Geometry: final body of the model. Coordinates: model frame, mm. Face numbers are marked on the shaded views. A direction names the side the tool comes from. Give positions to 0.01 mm unless a question says otherwise; leave off trailing zeros. Order: outer loops, then holes, each group sorted by start corner. A loop starts at its lowest first (then second) coordinate and runs counter-clockwise, first axis right, second up. Notation, with made-up numbers: (-9.75, -8) - (24.25, -8) arc R12 cw to (24.25, 0) - close; hole circle Ø9 at (13.25, 55.5). An arc over 180 degrees is marked (long way). Put each result on its own line as item: value. Start each with the question number.
1. Ray query, line 1 along Z through (x, y) = (-4, 16.5); line 2 along X through (y, z) = (12, -33); line 3 along X through (y, z) = (17, -17.5). Return the intervals inside material, ascending. Write a range as from..to.
2. Section A-A on x = 0. Return the cut outline in (y, z), plus the area to 3 significant figures.
3. Mould query, pull axis Z, two halves, no side actions, for the marked faces 5, 6 and 7. Classes: pulls with the +Z half, pulls with the -Z half, needs draft (parallel to the pull), parting line crosses it, or undercut.
4. First-contact query: P1, Ø3, axis at y = 14.5, z = -39, coming from the +X side; P2, Ø3.5, axis at y = 11, z = 25.59, coming from the -X side; P3, Ø6.5, axis at y = 8.5, z = 25, coming from the +X side. Flat tips, straight axial feed; report the tip coordinate or a pass-through.
5. Section B-B on z = 0. Return the cut outline in (x, y).
6. Set-up query: the marked faces 1, 2, 3 and 4. Return all of +Z, -Z, +X, -X, +Y, -Y with unobstructed straight access to the full face (end or side cutting, diameter ignored); none if empty.
7. Section C-C on y = 17.5. Return the cut outline in (x, z), plus the area to 3 significant figures.
8. Section D-D on y = 11. Count the separate pieces of the cut face and the enclosed holes in it, plus the area to 3 significant figures.
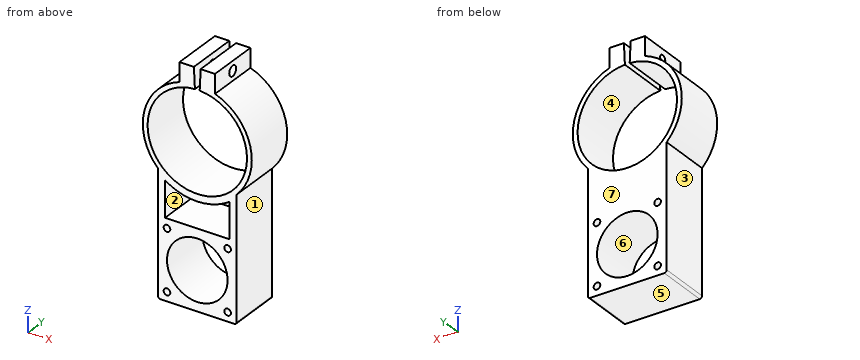
from build123d import *

# Parameters (mm, degrees)
BOSS_EXTRUDE1_DEPTH = 22
CUT_EXTRUDE1_REACH  = 79.458
SKETCH4_R           = 1.5875
CUT_EXTRUDE2_REACH  = 79.458
SKETCH5_R           = 2.159
SKETCH7_R           = 12.7
CUT_EXTRUDE3_DEPTH  = 75.871591195
SKETCH8_R           = 1.397
CUT_EXTRUDE4_DEPTH  = 75.871591195
CUT_EXTRUDE5_DEPTH  = 19
FILLET1_R           = 1


with BuildPart() as part:
    # Sketch1 → Boss-Extrude1 (new body)
    with BuildSketch(Plane(origin=(0, 0, 0), x_dir=(1, 0, 0), z_dir=(0, 1, 0))):
        with BuildLine():
            Line((1, -20.803980004), (1.422212938, -29.587689527))
            Line((1.422212938, -29.587689527), (7.422212938, -29.587689527))
            Line((7.422212938, -29.587689527), (7.422212938, -21.587689527))
            ThreePointArc((7.422212938, -21.587689527), (22.182667824, -5.389511316), (16.5, 15.775537519))
            Line((16.5, 15.775537519), (16.5, 67.828))
            Line((16.5, 67.828), (-16.5, 67.828))
            Line((-16.5, 67.828), (-16.5, 15.775537519))
            ThreePointArc((-16.5, 15.775537519), (-22.182667824, -5.389511316), (-7.422212938, -21.587689527))
            Line((-7.422212938, -21.587689527), (-7.422212938, -29.587689527))
            Line((-7.422212938, -29.587689527), (-1.422212938, -29.587689527))
            Line((-1.422212938, -29.587689527), (-1, -20.803980004))
            ThreePointArc((-1, -20.803980004), (0, 20.828), (1, -20.803980004))
        make_face()
    extrude(amount=BOSS_EXTRUDE1_DEPTH)

    # Cut-Extrude1: up to this plane
    cut_extrude1_end = Plane(origin=(-1, 22, 20.803980004), z_dir=(-0.9988467449508261, 0, -0.04801229114653368))
    # Sketch4 → Cut-Extrude1 (cut, up to the surface)
    with BuildSketch(Plane.ZY.offset(7.422212938), mode=Mode.PRIVATE) as cut_extrude1_sk1:
        with Locations((25.587689527, 11)):
            Circle(SKETCH4_R)
    cut_extrude1_tool1 = split(extrude(cut_extrude1_sk1.sketch, amount=-CUT_EXTRUDE1_REACH, mode=Mode.PRIVATE), bisect_by=cut_extrude1_end, keep=Keep.BOTH, mode=Mode.PRIVATE)
    add(cut_extrude1_tool1.solids().sort_by_distance((-7.422213, 11, 25.58769))[0], mode=Mode.SUBTRACT)

    # Cut-Extrude2: up to this plane
    cut_extrude2_end = Plane(origin=(1, 22, 20.803980004), z_dir=(0.9988467449508261, 0, -0.04801229114653392))
    # Sketch5 → Cut-Extrude2 (cut, up to the surface)
    with BuildSketch(Plane(origin=(7.422212938, 0, 0), x_dir=(0, 0, -1), z_dir=(1, 0, 0)), mode=Mode.PRIVATE) as cut_extrude2_sk1:
        with Locations((-25.587689527, 11)):
            Circle(SKETCH5_R)
    cut_extrude2_tool1 = split(extrude(cut_extrude2_sk1.sketch, amount=-CUT_EXTRUDE2_REACH, mode=Mode.PRIVATE), bisect_by=cut_extrude2_end, keep=Keep.BOTH, mode=Mode.PRIVATE)
    add(cut_extrude2_tool1.solids().sort_by_distance((7.422213, 11, 25.58769))[0], mode=Mode.SUBTRACT)

    # Sketch7 → Cut-Extrude3 (cut, through all)
    with BuildSketch(Plane.XZ):
        with Locations(Location((0, -51.328, 0), (0, 0, 270))):
            Circle(SKETCH7_R)
    extrude(amount=-CUT_EXTRUDE3_DEPTH, mode=Mode.SUBTRACT)

    # Sketch8 → Cut-Extrude4 (cut, through all)
    with BuildSketch(Plane(origin=(0, 22, 0), x_dir=(1, 0, 0), z_dir=(0, 1, 0))):
        with Locations(Location((12.7, 64.028, 0), (0, 0, 270))):
            Circle(SKETCH8_R)
        with Locations(Location((12.7, 38.628, 0), (0, 0, 270))):
            Circle(SKETCH8_R)
        with Locations(Location((-12.7, 38.628, 0), (0, 0, 270))):
            Circle(SKETCH8_R)
        with Locations(Location((-12.7, 64.028, 0), (0, 0, 270))):
            Circle(SKETCH8_R)
    extrude(amount=-CUT_EXTRUDE4_DEPTH, mode=Mode.SUBTRACT)

    # Sketch9 → Cut-Extrude5 (cut)
    with BuildSketch(Plane.XZ):
        with BuildLine():
            Line((-13.5, -34.628), (13.5, -34.628))
            Line((13.5, -34.628), (13.5, -19.634754493))
            ThreePointArc((13.5, -19.634754493), (0, -23.828), (-13.5, -19.634754493))
            Line((-13.5, -19.634754493), (-13.5, -34.628))
        make_face()
    extrude(amount=-CUT_EXTRUDE5_DEPTH, mode=Mode.SUBTRACT)

    # Fillet1
    fillet1_edges = [part.edges().sort_by_distance(p)[0] for p in [
        (-16.5, 11, -67.828),
        (16.5, 11, -67.828),
    ]]
    fillet(fillet1_edges, radius=FILLET1_R)


solid = part.part
Resolved:
1. line 1: -67.83..-63.38, -39.27..-34.63, -23.49..-20.44, 20.44..29.59
1. line 2: -16.5..-13.5, 13.5..16.5
1. line 3: -16.5..-11.29, 11.29..16.5
2. outline: (0, -67.83) - (22, -67.83) - (22, -64.03) - (0, -64.03) - close; (0, -38.63) - (22, -38.63) - (22, -20.83) - (0, -20.83) - (0, -23.83) - (19, -23.83) - (19, -34.63) - (0, -34.63) - close
2. area: 270 mm^2
3. face 5: pulls with the -Z half
3. face 6: undercut
3. face 7: needs draft
4. P1: x = 16.5
4. P2: x = -7.42
4. P3: x = 7.42
5. outline: (-22.83, 0) - (-20.83, 0) - (-20.83, 22) - (-22.83, 22) - close; (20.83, 0) - (22.83, 0) - (22.83, 22) - (20.83, 22) - close
6. face 1: -Z, +X, +Y, -Y
6. face 2: -Y
6. face 3: -Z, -X, +Y, -Y
6. face 4: +Y, -Y
7. outline: (-16.5, -66.83) arc R1 ccw to (-15.5, -67.83) - (15.5, -67.83) arc R1 ccw to (16.5, -66.83) - (16.5, -15.78) arc R22.83 ccw to (7.42, 21.59) - (7.42, 29.59) - (1.42, 29.59) - (1, 20.8) arc R20.83 cw (long way) to (-1, 20.8) - (-1.42, 29.59) - (-7.42, 29.59) - (-7.42, 21.59) arc R22.83 ccw to (-16.5, -15.78) - close; hole circle Ø2.79 at (-12.7, -64.03); hole circle Ø2.79 at (-12.7, -38.63); hole (-13.5, -34.63) - (13.5, -34.63) - (13.5, -19.63) arc R23.83 cw to (-13.5, -19.63) - close; hole circle Ø25.4 at (0, -51.33); hole circle Ø2.79 at (12.7, -64.03); hole circle Ø2.79 at (12.7, -38.63)
7. area: 1,060 mm^2
8. separate pieces: 3
8. enclosed holes: 6
8. area: 1,010 mm^2
